Part model, mm, in its own coordinate system. Face numbers are marked on the shaded views. Give positions to 0.01 mm unless a question says otherwise; leave off trailing zeros. Write each loop counter-clockwise with the first axis right and the second up, starting at its lowest first coordinate (ties: lowest second). Pieces come first, ordered by that corner, then holes. Notation, with made-up numbers: M 89,79 L 139,79 A13 cw 139,91 Z; hole C 83,57 d11. An arc over 180 degrees is marked long. Use a Markdown table: item, result.
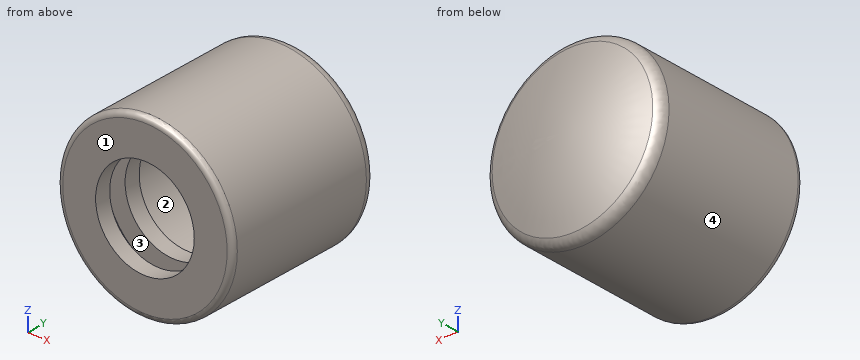
```python
from build123d import *

# Parameters (mm, degrees)
CONG_1_R = 2
CONG_2_R = 1


with BuildPart() as part:
    # Esquisse1 → Révolution1 (revolve)
    with BuildSketch(Plane.XY, mode=Mode.PRIVATE) as r_volution1_sk:
        with BuildLine():
            Line((0, 31.9), (0, 28.9))
            Line((0, 28.9), (-12.5, 28.9))
            Line((-12.5, 28.9), (-12.5, 12.6))
            Line((-12.5, 12.6), (-12.5, 9.3))
            Line((-12.5, 9.3), (-9, 9.3))
            Line((-9, 9.3), (-9, 6.3))
            Line((-9, 6.3), (-12.5, 6.3))
            Line((-12.5, 6.3), (-12.5, 3))
            Line((-12.5, 3), (-9, 3))
            Line((-9, 3), (-9, 0))
            Line((-9, 0), (-12.5, 0))
            Line((-12.5, 0), (-16, 0))
            Line((-16, 0), (-16, 29.95948169))
            ThreePointArc((-16, 29.95948169), (-8.133981927, 32.158765663), (0, 32.9))
            Line((0, 32.9), (0, 31.9))
        make_face()
    revolve(r_volution1_sk.sketch.rotate(Axis((0, 0, 0), (0, 1, 0)), 180), axis=Axis((0, 0, 0), (0, 1, 0)))

    # Congé1
    cong_1_edges = [part.edges().sort_by_distance(p)[0] for p in [
        (-16, 29.95948169, 0),
    ]]
    fillet(cong_1_edges, radius=CONG_1_R)

    # Congé2
    cong_2_edges = [part.edges().sort_by_distance(p)[0] for p in [
        (-16, 0, 0),
    ]]
    fillet(cong_2_edges, radius=CONG_2_R)


solid = part.part
```
1. Two-plate mould, pull along Y, no slides. Class the marked faces 1, 2, 3 and 4: released by +Y, released by -Y, zero draft, split by the parting line, or undercut.
Findings below:
| item | result |
|---|---|
| face 1 | released by -Y |
| face 2 | undercut |
| face 3 | undercut |
| face 4 | zero draft |
2. Cut at B-B, the plane z = 11.5. State how many separate pieces and enclosed holes the cut face has, then the cut area to 3 significant figures.
Findings below:
| item | result |
|---|---|
| separate pieces | 1 |
| enclosed holes | 2 |
| area | 462 mm2 |
3. Cut at A-A, the plane y = 25. Give the cut face in (x, z), then the cut area to 3 significant figures.
Findings below:
| item | result |
|---|---|
| outline | C 0,0 d32; hole C 0,0 d25 |
| area | 313 mm2 |
4. Drill centre lines: L1, parallel to Z at x = 0, y = 7.7; L2, parallel to X at y = 20, z = 6.5; L3, parallel to Z at x = 0, y = 4.35. Where is each one in solid material? Low to high.
Findings below:
| item | result |
|---|---|
| L1 | -16 to -9, 9 to 16 |
| L2 | -14.62 to -10.68, 10.68 to 14.62 |
| L3 | -16 to -12.5, 12.5 to 16 |
5. Drop flat-ended pins along their axis: P1, Ø7.5, axis at x = -5, z = 2, coming from the +Y side; P2, Ø1.5, axis at x = 8, y = 22.5, coming from the -Z side; P3, Ø15, axis at x = 0, z = 0, coming from the -Y side. Give the stop position or say it passes through.
Findings below:
| item | result |
|---|---|
| P1 | y = 32.87 |
| P2 | z = -14.26 |
| P3 | y = 28.9 |
